Autodesk Inventor part; units mm, degrees
ref_plane "YZ Plane" through (0, 0, 0) normal (1, 0, 0) x (0, 1, 0)
ref_plane "XZ Plane" through (0, 0, 0) normal (0, 1, 0) x (-1, 0, 0)
ref_plane "XY Plane" through (0, 0, 0) normal (0, 0, 1) x (1, 0, 0)
sketch "Sketch1" plane through (0, 0, 0) normal (0, 0, 1) x (1, 0, 0)
  line L0 (0, 0) -> (-5, 0)
  line L1 (0, 0) -> (0, 5)
  line L2 (0, 5) -> (5, 5)
  line L3 (5, 5) -> (5, 45)
  line L4 (5, 45) -> (10, 45)
  line L5 (10, 45) -> (10, 47.5)
  line L6 (5, 52.5) -> (0, 52.5)
  line L7 (-5, 47.5) -> (-5, 0)
  line L8 (0, 0) -> (10, 0)
  line L9 (10, 0) -> (10, -5)
  line L10 (10, -5) -> (-5, -5)
  line L11 (-5, -5) -> (-5, 0)
  arc A0 (10, 47.5) -> (5, 52.5) centre (5, 47.5) ccw
  arc A1 (0, 52.5) -> (-5, 47.5) centre (0, 47.5) ccw
  point P0 (10, 52.5)
  point P1 (-5, 52.5)
  dimension "d0" = 5
  dimension "d1" = 5
  dimension "d2" = 5
  dimension "d3" = 40
  dimension "d4" = 5
  dimension "d5" = 7.5
  dimension "d8" = 10
  dimension "d9" = 5
  dimension "d10" = 5
extrude "Extrusion1" add sketch "Sketch1" along normal blind 6.5
properties part number "block"
CAD build for the part. Positions are in the model's coordinates, mm. A direction names the side the tool comes from. Coordinates: 2 decimals unless noted, no trailing zeros. Order: outer loops, then holes, each group sorted by start corner. A loop starts at its lowest first (then second) coordinate and runs counter-clockwise, first axis right, second up.
(1) Mould opens along Y. For faces 3 (the face through (-3.57, 51, 3.2)), 4 (the face through (5, 25, 3)), 5 (the face through (1, 24, 0)), 6 (the face through (5, 0, 3)) say: released by +Y, released by -Y, zero draft, split by the parting line, or undercut.
Solution:
face 3: released by +Y
face 4: undercut
face 5: zero draft
face 6: undercut
(2) Which spindle directions (+Z, -Z, +X, -X, +Y, -Y) get a long thin tool onto all of the face, cutting with end or side? Do faces 1 (the face through (8.5, 51.07, 3.2)), 2 (the face through (7, 45, 3)). Say none if no direction does.
Solution:
face 1: +Z, -Z, +X, +Y
face 2: +Z, -Z, +X
(3) Drill centre lines: L1, parallel to Y at x = 2.25, z = 3; L2, parallel to X at y = 17, z = 2.25; L3, parallel to X at y = 3, z = 6. Where is each one in solid material? Low to high.
Solution:
L1: y = -5 to 0, 5 to 52.5
L2: x = -5 to 5
L3: x = -5 to 0
(4) Saw through at C-C, the plane x = 2.5. Write the cut outline in (y, z), and give its area (3 significant figures).
Solution:
outline: (-5, 0) - (0, 0) - (0, 6.5) - (-5, 6.5) - close; (5, 0) - (52.5, 0) - (52.5, 6.5) - (5, 6.5) - close
area: 341 mm2
(5) Saw through at D-D, the plane y = 21. Write the cut outline in (x, z).
Solution:
outline: (-5, 0) - (5, 0) - (5, 6.5) - (-5, 6.5) - close
(6) Saw through at B-B, the plane z = 4. Write the cut outline in (x, y).
Solution:
outline: (-5, -5) - (10, -5) - (10, 0) - (0, 0) - (0, 5) - (5, 5) - (5, 45) - (10, 45) - (10, 47.5) arc R5 ccw to (5, 52.5) - (0, 52.5) arc R5 ccw to (-5, 47.5) - close
(7) Saw through at A-A, the plane x = 5.5. Write the cut outline in (y, z).
Solution:
outline: (-5, 0) - (0, 0) - (0, 6.5) - (-5, 6.5) - close; (45, 0) - (52.47, 0) - (52.47, 6.5) - (45, 6.5) - close
(8) Pin check, flat tips, straight feed: pin 1 Ø2 at (x, y) = (7.5, 4.5) entering from -Z; pin 2 Ø3 at (y, z) = (25, 2.5) entering from +X. Stop position of each tip, or through.
Solution:
pin 1: passes through
pin 2: stops at x = 5
